The listing builds one solid part. Answer for the finished solid, in the listing's coordinates (mm). A direction names the side the tool comes from. Round coordinates to 2 decimals unless told otherwise and drop trailing zeros. Write each loop counter-clockwise with the first axis right and the second up, starting at its lowest first coordinate (ties: lowest second). Pieces come first, ordered by that corner, then holes.
from build123d import *

# Parameters (mm, degrees)
F0_R     = 31.75
F1_DEPTH = 127
F2_R     = 31.75
F3_DEPTH = 30.48
F4_SIZE  = 30.48
F5_R     = 14.175594
F6_DEPTH = 25.4


with BuildPart() as f1:
    # F0 (on Top) → F1 (new body)
    with BuildSketch(Plane.XY):
        Circle(F0_R)
    extrude(amount=F1_DEPTH)

    # F2 (on face) → F3 (join)
    with BuildSketch(Plane.XY.offset(127)):
        Circle(F2_R)
    extrude(amount=F3_DEPTH)

    # F4
    f4_edges = [f1.edges().sort_by_distance(p)[0] for p in [
        (-31.75, 0, 157.48),
    ]]
    chamfer(f4_edges, length=F4_SIZE)

    # F5 (on face) → F6 (join)
    with BuildSketch(Plane(origin=(0, 0, 0), x_dir=(1, 0, 0), z_dir=(0, 0, -1))):
        Circle(F5_R)
    extrude(amount=F6_DEPTH)


solid = f1.part
1. Straight lines are drawn through the part: line 1 along Y through (x, z) = (-28, 108); line 2 along Y through (x, z) = (-21, 89); line 3 along Z through (x, y) = (26, -17.5). For each, find the intervals that lie inside material, in ascending order.
Geometry says:
line 1: y = -14.97 to 14.97
line 2: y = -23.81 to 23.81
line 3: z = 0 to 127.41
2. Given pin 1 (2 mm diameter, centred on x = 13.5, z = 39, fed in from -Y); pin 2 (4 mm diameter, centred on x = -23, y = 17, fed in from +Z); pin 3 (4 mm diameter, centred on x = -22, y = 21, fed in from +Z), each flat-ended and moving along its own axis, determine where each tip first touches the part or whether it passes through.
Geometry says:
pin 1: stops at y = -29.19
pin 2: stops at z = 132.15
pin 3: stops at z = 130.34
3. A tool of negligible diameter and unlimited length cuts with its end or side. For faces 1 (the face through (0, 0, -25.4)), 2 (the face through (-3.07, 13.84, -12.52)), from which of +Z, -Z, +X, -X, +Y, -Y can it reach the whole face along a straight path? Write none if from no direction.
Geometry says:
face 1: -Z, +X, -X, +Y, -Y
face 2: -Z
4. Section A-A on z = 76 is taken. Determine the outline of the cut face in (x, y), plus the area to 3 significant figures.
Geometry says:
outline: circle Ø63.5 at (0, 0)
area: 3,170 mm2
